For this review, take the finished solid that the model builds, in its own axes (mm). A direction names the side the tool comes from. Coordinates: 2 decimals unless noted, no trailing zeros. Write each loop counter-clockwise with the first axis right and the second up, starting at its lowest first coordinate (ties: lowest second). Pieces come first, ordered by that corner, then holes.
```python
from build123d import *

# Parameters (mm, degrees)
DAMPINGBRACKETGEOMETRY_DEPTH                    = 50
CSK_FOR_M3_FLAT_HEAD_MACHINE_SCREW1_D           = 3.4
CSK_FOR_M3_FLAT_HEAD_MACHINE_SCREW1_CSINK_D     = 6.3
CSK_FOR_M3_FLAT_HEAD_MACHINE_SCREW1_CSINK_ANGLE = 90
SKETCH5_W                                       = 13.75
SKETCH5_H                                       = 23.30481037
CUT_EXTRUDE1_DEPTH                              = 72.15904504
FILLET1_R                                       = 5


with BuildPart() as part:
    # Sketch1 → DampingBracketGeometry (new body)
    with BuildSketch(Plane.XY):
        Polygon((10.886169422, 19.440829014), (30.820361381, 19.440829014), (39.465737075, 16.294169597), (40.149777362, 18.173554838), (30.752851154, 21.593756272), (37.593254021, 40.387608687), (46.990180228, 36.967407254), (47.674220515, 38.846792496), (35.458216445, 43.293054359), (29.251713991, 26.240829014), (10.886169422, 26.240829014), (10.886169422, 24.940829014), (25.886169422, 24.940829014), (25.886169422, 21.640829014), (10.886169422, 21.640829014), align=None)
    extrude(amount=DAMPINGBRACKETGEOMETRY_DEPTH)

    # CSK for M3 Flat Head Machine Screw1 (through all)
    with Locations(Plane(origin=(0, 26.240829014, 0), x_dir=(1, 0, 0), z_dir=(0, 1, 0))):
        with Locations((21.136169422, -8), (21.136169422, -42)):
            CounterSinkHole(CSK_FOR_M3_FLAT_HEAD_MACHINE_SCREW1_D / 2, CSK_FOR_M3_FLAT_HEAD_MACHINE_SCREW1_CSINK_D / 2, counter_sink_angle=CSK_FOR_M3_FLAT_HEAD_MACHINE_SCREW1_CSINK_ANGLE)

    # Sketch5 → Cut-Extrude1 (cut, through all)
    with BuildSketch(Plane(origin=(0, 26.240829014, 0), x_dir=(1, 0, 0), z_dir=(0, 1, 0))):
        with Locations((10.886169422, -25)):
            Rectangle(SKETCH5_W, SKETCH5_H)
    extrude(amount=-CUT_EXTRUDE1_DEPTH, mode=Mode.SUBTRACT)

    # Fillet1
    fillet1_edges = [part.edges().sort_by_distance(p)[0] for p in [
        (17.761169422, 20.540829014, 13.347594815),
        (17.761169422, 25.590829014, 13.347594815),
        (17.761169422, 25.590829014, 36.652405185),
        (17.761169422, 20.540829014, 36.652405185),
    ]]
    fillet(fillet1_edges, radius=FILLET1_R)


solid = part.part
```
1) Consider section D-D (y = 23). Give the boundary of the cut face in (x, z).
2) Tool access review of faces 1 (the face through (22, 26.241, 25)), 2 (the face through (17.761, 26, 25)), 3 (the face through (20, 21.641, 25)), 4 (the face through (23, 19.441, 25)), 5 (the face through (35.52, 19.86, 24.65)): name each direction out of +Z, -Z, +X, -X, +Y, -Y from which nothing blocks a thin tool from reaching the whole face with its end or side.
3) Consider section B-B (x = 15). Give the boundary of the cut face in (y, z).
4) Clearance check with flat-ended pins moving along their axes: P1, Ø2.5, axis at y = 24, z = 36, coming from the -X side; P2, Ø1.5, axis at y = 28, z = 18, coming from the -X side; P3, Ø1, axis at y = 25.5, z = 24.5, coming from the -X side; P4, Ø12, axis at x = 19, z = 35, coming from the +Y side. State where each tip first meets the part, or that it passes through.
5) The part is to be moulded in two halves that separate along Z. For faces 6 (the face through (20, 24.941, 25)), 7 (the face through (19.566, 20.525, 8.651)), 8 (the face through (31, 28, 50)), say which applies: pulls with the +Z half, pulls with the -Z half, needs draft (parallel to the pull), parting line crosses it, or undercut.
6) For L1, parallel to Y at x = 18, z = 43.5; L2, parallel to Z at x = 23.5, y = 26; L3, parallel to X at y = 28, z = 40, list the stretches that pass through material, from the lowest coordinate up.
7) Consider section C-C (z = 8). Give the boundary of the cut face in (x, y), then the cut area to 3 significant figures.
8) Consider section A-A (z = 27.5). Give the boundary of the cut face in (x, y), then the cut area to 3 significant figures.
Results:
1. outline: (25.89, 0) - (31.26, 0) - (31.26, 50) - (25.89, 50) - close
2. face 1: +Z, -Z, -X, +Y
2. face 2: -X, +Y, -Y
2. face 3: +Z, -Z, -X
2. face 4: +Z, -Z, -X, -Y
2. face 5: +Z, -Z, +X
3. outline: (19.44, 0) - (21.64, 0) - (21.64, 13.88) - (19.44, 13.88) - close; (19.44, 36.12) - (21.64, 36.12) - (21.64, 50) - (19.44, 50) - close; (24.94, 0) - (26.24, 0) - (26.24, 13.88) - (24.94, 13.88) - close; (24.94, 36.12) - (26.24, 36.12) - (26.24, 50) - (24.94, 50) - close
4. P1: stops at x = 10.89
4. P2: stops at x = 29.62
4. P3: stops at x = 17.76
4. P4: stops at y = 26.24
5. face 6: needs draft
5. face 7: undercut
5. face 8: pulls with the +Z half
6. L1: y = 19.44 to 21.64, 24.94 to 26.24
6. L2: z = 0 to 6.3, 9.7 to 40.3, 43.7 to 50
6. L3: x = 29.89 to 33.08
7. outline: (10.89, 19.44) - (19.44, 19.44) - (19.44, 21.64) - (10.89, 21.64) - close; (10.89, 24.94) - (19.29, 24.94) - (17.99, 26.24) - (10.89, 26.24) - close; (22.84, 19.44) - (30.82, 19.44) - (39.47, 16.29) - (40.15, 18.17) - (30.75, 21.59) - (37.59, 40.39) - (46.99, 36.97) - (47.67, 38.85) - (35.46, 43.29) - (29.25, 26.24) - (24.29, 26.24) - (22.99, 24.94) - (25.89, 24.94) - (25.89, 21.64) - (22.84, 21.64) - close
7. area: 168 mm2
8. outline: (17.76, 19.44) - (30.82, 19.44) - (39.47, 16.29) - (40.15, 18.17) - (30.75, 21.59) - (37.59, 40.39) - (46.99, 36.97) - (47.67, 38.85) - (35.46, 43.29) - (29.25, 26.24) - (17.76, 26.24) - (17.76, 24.94) - (25.89, 24.94) - (25.89, 21.64) - (17.76, 21.64) - close
8. area: 158 mm2
